from build123d import *

# Parameters (mm, degrees)
SKETCH1_R           = 15
BOSS_EXTRUDE1_DEPTH = 5
FILLET1_R           = 3
SKETCH2_R           = 1.8
CUT_EXTRUDE1_DEPTH  = 2.2


with BuildPart() as part:
    # Sketch1 → Boss-Extrude1 (new body)
    with BuildSketch(Plane.XY):
        Circle(SKETCH1_R)
    extrude(amount=BOSS_EXTRUDE1_DEPTH)

    # Fillet1
    fillet1_edges = [part.edges().sort_by_distance(p)[0] for p in [
        (-15, 0, 5),
    ]]
    fillet(fillet1_edges, radius=FILLET1_R)

    # Sketch2 → Cut-Extrude1 (cut)
    with BuildSketch(Plane(origin=(0, 0, 0), x_dir=(-1, 0, 0), z_dir=(0, 0, -1))):
        Circle(SKETCH2_R)
    extrude(amount=-CUT_EXTRUDE1_DEPTH, mode=Mode.SUBTRACT)


solid = part.part
CAD build for the part. Positions are in the model's coordinates, mm. A direction names the side the tool comes from. Coordinates: 2 decimals unless noted, no trailing zeros. Loops run counter-clockwise (first coordinate to the right, second up) from the corner with the lowest first, then second, coordinate; pieces in that order, holes last. Notation, with made-up numbers: (-10, 43) - (15, 43) arc R12 ccw to (15, 65) - close; hole circle Ø8 at (35, 13.25). An arc over 180 degrees is marked (long way). Write item = value, one per line. Start each with the question number.
Q1. Pull direction X, two halves, no side cores. Call faces 3 (the cylindrical face through (-1.717, 0.541, 1.085)), 4 (the cylindrical face through (-14.985, 0.66, 0.986)), 5 (the flat face through (0, 0, 5)): pulls with the +X half, pulls with the -X half, needs draft (parallel to the pull), parting line crosses it, or undercut.
Q2. Flat gauge pins, fed straight in: pin 1 Ø3 at (x, y) = (0, 0) entering from -Z; pin 2 Ø2 at (y, z) = (2, 3) entering from +X. Where does each tip first touch, or does it go through?
Q3. Which spindle directions (+Z, -Z, +X, -X, +Y, -Y) get a long thin tool onto all of the face, cutting with end or side? Do faces 1 (the flat face through (3, 0, 0)), 2 (the flat face through (0, 0, 2.2)). Say none if no direction does.
Q4. Drill centre lines: L1, parallel to Y at x = 0, z = 1.3; L2, parallel to Y at x = -4.25, z = 0.5; L3, parallel to Y at x = 3.5, z = 3.2. Where is each one in solid material? Low to high.
Q5. Cut at C-C, the plane z = 4.15. List the corners of the cut face in (x, y).
Q6. Cut at A-A, the plane y = 0. List the corners of the cut face in (x, z).
Computed:
q1.face_3 = undercut
q1.face_4 = parting line crosses it
q1.face_5 = needs draft
q2.pin_1 = 2.2
q2.pin_2 = 14.93
q3.face_1 = -Z, +X, -X, +Y, -Y
q3.face_2 = -Z
q4.L1 = -15 to -1.8, 1.8 to 15
q4.L2 = -14.39 to 14.39
q4.L3 = -14.33 to 14.33
q5.outline = circle Ø28.18 at (0, 0)
q6.outline = (-15, 0) - (-1.8, 0) - (-1.8, 2.2) - (1.8, 2.2) - (1.8, 0) - (15, 0) - (15, 2) arc R3 ccw to (12, 5) - (-12, 5) arc R3 ccw to (-15, 2) - close
